Build history of the part. All positions in model axes, mm. A direction names the side the tool comes from. Round coordinates to 2 decimals unless told otherwise and drop trailing zeros. Loops run counter-clockwise (first coordinate to the right, second up) from the corner with the lowest first, then second, coordinate; pieces in that order, holes last. Notation, with made-up numbers: (83.25, 75) - (132.25, 75) arc R12 cw to (132.25, 90) - close; hole circle Ø5 at (54.25, 89). An arc over 180 degrees is marked (long way). Use a Markdown table: item, result.
from build123d import *

# Parameters (mm, degrees)
F1_DEPTH = 25.4
F2_W     = 31.75
F2_H     = 12.7
F2_W_2   = 88.9
F2_R     = 15.875
F3_DEPTH = 25.401
F4_R     = 6.34999
F5_SIZE  = 12.7


# Not quite as in the source:
# - a fillet or chamfer is up to 0.001 mm smaller than in the source, because OpenCascade refuses the exact size


with BuildPart() as f1:
    # F0 (on Top) → F1 (new body)
    with BuildSketch(Plane.XY):
        Polygon((-50.9642694569, 222.8586515407), (-409.1042694569, 222.8586515407), (-409.1042694569, 57.7525011744), (-409.1042694569, 32.4011304667), (-409.1042694569, -132.7413484593), (196.6857305431, -132.7413484593), (291.9357305431, -56.5413484593), (291.9357305431, 222.8586515407), (-49.417052418, 222.8586515407), align=None)
    extrude(amount=F1_DEPTH)

    # F2 (on face) → F3 (cut, through all)
    with BuildSketch(Plane.XY.offset(25.4)):
        with Locations((-393.2292694569, 45.0586515407)):
            Rectangle(F2_W, F2_H)
        with Locations((181.4457305431, 45.0586515407)):
            Rectangle(F2_W_2, F2_H)
        with BuildLine():
            Line((-59.8542694569, -142.5310963776), (-59.8542694569, -94.6413484593))
            ThreePointArc((-59.8542694569, -94.6413484593), (-66.2042694569, -88.2913484593), (-72.5542694569, -94.6413484593))
            Line((-72.5542694569, -94.6413484593), (-72.5542694569, -137.446552515))
            Line((-72.5542694569, -137.446552515), (-59.8542694569, -142.5310963776))
        make_face()
        with Locations((-66.2042694569, 184.7586515407)):
            Circle(F2_R)
    extrude(amount=-F3_DEPTH, mode=Mode.SUBTRACT)

    # F4 (radius 6.35 in the source; OpenCascade refuses exactly that, so slightly less here)
    f4_edges = [f1.edges().sort_by_distance(p)[0] for p in [
        (-377.354269, 51.408652, 12.7),
        (225.895731, 51.408652, 12.7),
        (225.895731, 38.708652, 12.7),
        (-377.354269, 38.708652, 12.7),
        (136.995731, 51.408652, 12.7),
        (136.995731, 38.708652, 12.7),
    ]]
    fillet(f4_edges, radius=F4_R)

    # F5
    f5_edges = [f1.edges().sort_by_distance(p)[0] for p in [
        (291.935731, 83.158652, 0),
    ]]
    chamfer(f5_edges, length=F5_SIZE)


solid = f1.part
Q1. Cut at A-A, the plane y = -105. List the corners of the cut face in (x, z), plus the area to 3 significant figures.
Results found:
| item | result |
|---|---|
| outline | (-409.1, 0) - (-72.55, 0) - (-72.55, 25.4) - (-409.1, 25.4) - close; (-59.85, 0) - (231.36, 0) - (231.36, 25.4) - (-59.85, 25.4) - close |
| area | 15,900 mm2 |
Q2. Drop flat-ended pins along their axis: pin 1 (7.5 mm diameter, centred on y = -122.5, z = 7, fed in from +X); pin 2 (1.5 mm diameter, centred on y = -57.5, z = 4, fed in from +X). Give the stop position or say it passes through.
Results found:
| item | result |
|---|---|
| pin 1 | stops at x = 214.17 |
| pin 2 | stops at x = 283.99 |
Q3. Pull direction X, two halves, no side cores. Call faces 5 (the face through (285.675, 76.052, 6.439)), 6 (the face through (-409.104, 138, 13)), 7 (the face through (-69.646, 169.261, 12.878)): pulls with the +X half, pulls with the -X half, needs draft (parallel to the pull), parting line crosses it, or undercut.
Results found:
| item | result |
|---|---|
| face 5 | pulls with the +X half |
| face 6 | pulls with the -X half |
| face 7 | undercut |
Q4. Probe line 1 (Y direction, x = 193, z = 1.25); line 2 (X direction, y = -110.5, z = 16.75); line 3 (X direction, y = 41, z = 22.5). List the from-to ranges inside material, lowest first.
Results found:
| item | result |
|---|---|
| line 1 | y = -132.74 to 38.71, 51.41 to 222.86 |
| line 2 | x = -409.1 to -72.55, -59.85 to 224.49 |
| line 3 | x = -378.82 to 138.46, 224.43 to 291.94 |
Q5. Which spindle directions (+Z, -Z, +X, -X, +Y, -Y) get a long thin tool onto all of the face, cutting with end or side? Do faces 1 (the face through (-397, 38.709, 13)), 2 (the face through (181, 51.409, 13)), 3 (the face through (291.936, 81, 19)), 4 (the face through (-59.854, -114, 13)). Say none if no direction does.
Results found:
| item | result |
|---|---|
| face 1 | +Z, -Z, -X |
| face 2 | +Z, -Z |
| face 3 | +Z, -Z, +X, +Y, -Y |
| face 4 | +Z, -Z, -Y |
Q6. Cut at B-B, the plane z = 17. Count the separate pieces of the cut face and the enclosed holes in it, plus the area to 3 significant figures.
Results found:
| item | result |
|---|---|
| separate pieces | 1 |
| enclosed holes | 2 |
| area | 243,000 mm2 |
Q7. Cut at C-C, the plane x = 235.5. List the corners of the cut face in (y, z).
Results found:
| item | result |
|---|---|
| outline | (-101.69, 0) - (222.86, 0) - (222.86, 25.4) - (-101.69, 25.4) - close |
